CAD build for the part. Positions are in the model's coordinates, mm. Round coordinates to 2 decimals unless told otherwise and drop trailing zeros. Write each loop counter-clockwise with the first axis right and the second up, starting at its lowest first coordinate (ties: lowest second). Pieces come first, ordered by that corner, then holes. Notation, with made-up numbers: (18.25, 59) - (54.25, 59) arc R22 ccw to (54.25, 79) - close; hole circle Ø7 at (50.25, 9). An arc over 180 degrees is marked (long way). Answer in a Markdown table with one row per item.
```python
from build123d import *

# Parameters (mm, degrees)
SKETCH_3_R        = 1.65
EXTRUDE_242_DEPTH = 2
CHAMFER_C1_SIZE   = 1


with BuildPart() as part:
    # 草图3 → Extrude 242 (new body)
    with BuildSketch(Plane.XY):
        Polygon((-31, -60), (31, -60), (36, -50), (38, -45), (38, 50), (28, 66), (-28, 66), (-38, 50), (-38, -45), (-36, -50), align=None)
        with Locations((-22, -56)):
            Circle(SKETCH_3_R, mode=Mode.SUBTRACT)
        with Locations((-25, 53)):
            Circle(SKETCH_3_R, mode=Mode.SUBTRACT)
        with Locations((-34, -43)):
            Circle(SKETCH_3_R, mode=Mode.SUBTRACT)
        with Locations((-34, 43)):
            Circle(SKETCH_3_R, mode=Mode.SUBTRACT)
        with Locations((22, -56)):
            Circle(SKETCH_3_R, mode=Mode.SUBTRACT)
        with Locations((25, 53)):
            Circle(SKETCH_3_R, mode=Mode.SUBTRACT)
        with Locations((34, -43)):
            Circle(SKETCH_3_R, mode=Mode.SUBTRACT)
        with Locations((34, 43)):
            Circle(SKETCH_3_R, mode=Mode.SUBTRACT)
    extrude(amount=EXTRUDE_242_DEPTH)

    # 底盖全周向心倒角_C1
    # the kernel refuses this chamfer: 1 mm, written as the material it takes off along each edge
    with BuildSketch(Plane(origin=(-38.955099084, -42.612252289, 0), x_dir=(-0.02552928052838921, -0.010211712211355682, 0.9996219169112968), z_dir=(0.3713906763541037, -0.9284766908852594, 0)), Plane(origin=(35.044900916, -52.387747711, 0), x_dir=(0.025529280528384445, -0.010211712211353776, 0.9996219169112968), z_dir=(0.3713906763541037, 0.9284766908852594, 0))) as chamfer_c1_piece_1:
        Polygon((CHAMFER_C1_SIZE * 0.999621916911, -CHAMFER_C1_SIZE * 0.0274958766106), (-CHAMFER_C1_SIZE * 0.0274958766106, -CHAMFER_C1_SIZE * 0.999621916911), (0, 0), align=None)
    extrude(amount=10.528530783, mode=Mode.SUBTRACT)
    with BuildSketch(Plane(origin=(-38, 52.571682988, 0), x_dir=(-0.02749587661058908, 0, 0.9996219169112968), z_dir=(0, -1, 0)), Plane(origin=(38, -47.571682988, 0), x_dir=(0.02749587661058908, 0, 0.9996219169112968), z_dir=(0, 1, 0))) as chamfer_c1_piece_2:
        Polygon((CHAMFER_C1_SIZE * 0.999621916911, -CHAMFER_C1_SIZE * 0.0274958766106), (-CHAMFER_C1_SIZE * 0.0274958766106, -CHAMFER_C1_SIZE * 0.999621916911), (0, 0), align=None)
    extrude(amount=100.143365976, mode=Mode.SUBTRACT)
    with BuildSketch(Plane(origin=(-26.637010742, 68.180782812, 0), x_dir=(-0.023316456732911925, 0.014572785458069957, 0.9996219169112968), z_dir=(-0.52999894000318, -0.847998304005088, 0)), Plane(origin=(39.362989258, 47.819217188, 0), x_dir=(0.023316456732909444, 0.014572785458068402, 0.9996219169112968), z_dir=(-0.52999894000318, 0.847998304005088, 0))) as chamfer_c1_piece_3:
        Polygon((CHAMFER_C1_SIZE * 0.999621916911, -CHAMFER_C1_SIZE * 0.0274958766106), (-CHAMFER_C1_SIZE * 0.0274958766106, -CHAMFER_C1_SIZE * 0.999621916911), (0, 0), align=None)
    extrude(amount=24.01132824, mode=Mode.SUBTRACT)
    with BuildSketch(Plane(origin=(30.571682988, 66, 0), x_dir=(0, 0.027495876610582174, 0.9996219169112968), z_dir=(-1, 0, 0))) as chamfer_c1_piece_4:
        Polygon((CHAMFER_C1_SIZE * 0.999621916911, -CHAMFER_C1_SIZE * 0.0274958766106), (-CHAMFER_C1_SIZE * 0.0274958766106, -CHAMFER_C1_SIZE * 0.999621916911), (0, 0), align=None)
    extrude(amount=61.143365976, mode=Mode.SUBTRACT)
    with BuildSketch(Plane(origin=(29.849908404, -62.300183191, 0), x_dir=(0.02459305968088644, -0.01229652984044322, 0.9996219169112968), z_dir=(0.447213595499958, 0.894427190999916, 0)), Plane(origin=(-37.150091596, -47.699816809, 0), x_dir=(-0.024593059680886434, -0.012296529840443217, 0.9996219169112968), z_dir=(0.447213595499958, -0.894427190999916, 0))) as chamfer_c1_piece_5:
        Polygon((CHAMFER_C1_SIZE * 0.999621916911, -CHAMFER_C1_SIZE * 0.0274958766106), (-CHAMFER_C1_SIZE * 0.0274958766106, -CHAMFER_C1_SIZE * 0.999621916911), (0, 0), align=None)
    extrude(amount=16.323705863, mode=Mode.SUBTRACT)
    with BuildSketch(Plane(origin=(-33.571682988, -60, 0), x_dir=(0, -0.02749587661058908, 0.9996219169112968), z_dir=(1, 0, 0))) as chamfer_c1_piece_6:
        Polygon((CHAMFER_C1_SIZE * 0.999621916911, -CHAMFER_C1_SIZE * 0.0274958766106), (-CHAMFER_C1_SIZE * 0.0274958766106, -CHAMFER_C1_SIZE * 0.999621916911), (0, 0), align=None)
    extrude(amount=67.143365976, mode=Mode.SUBTRACT)


solid = part.part
```
Q1. Saw through at A-A on x = -22. List the corners of the cut face in (y, z).
Computed:
| item | result |
|---|---|
| outline | (-60, 1) - (-59, 0) - (-57.65, 0) - (-57.65, 2) - (-60, 2) - close; (-54.35, 0) - (65, 0) - (66, 1) - (66, 2) - (-54.35, 2) - close |
Q2. Flat gauge pin, fed straight in: pin 1 (2 mm diameter, centred on x = -22, y = -56, fed in from -Z). Where does the tip first touch, or does it go through?
Computed:
| item | result |
|---|---|
| pin 1 | passes through |
Q3. Drill centre lines: line 1 (Y direction, x = 23.5, z = 0.25); line 2 (Y direction, x = -25, z = 1); line 3 (Y direction, x = -24, z = 0.8). Where is each one in solid material? Low to high.
Computed:
| item | result |
|---|---|
| line 1 | y = -59.25 to -56.69, -55.31 to 52.31, 53.69 to 65.25 |
| line 2 | y = -60 to 51.35, 54.65 to 66 |
| line 3 | y = -59.8 to 51.69, 54.31 to 65.8 |
Q4. Saw through at B-B on y = 43. List the corners of the cut face in (x, z).
Computed:
| item | result |
|---|---|
| outline | (-38, 1) - (-37, 0) - (-35.65, 0) - (-35.65, 2) - (-38, 2) - close; (-32.35, 0) - (32.35, 0) - (32.35, 2) - (-32.35, 2) - close; (35.65, 0) - (37, 0) - (38, 1) - (38, 2) - (35.65, 2) - close |
Q5. Saw through at D-D on y = -56. List the corners of the cut face in (x, z).
Computed:
| item | result |
|---|---|
| outline | (-33, 1) - (-31.88, 0) - (-23.65, 0) - (-23.65, 2) - (-33, 2) - close; (-20.35, 0) - (20.35, 0) - (20.35, 2) - (-20.35, 2) - close; (23.65, 0) - (31.88, 0) - (33, 1) - (33, 2) - (23.65, 2) - close |
Q6. Pull direction X, two halves, no side cores. Call faces 1 (the cylindrical face through (-26.65, 53.07, 0.99)), 2 (the flat face through (33.465, -55.07, 1.493)), 3 (the flat face through (-32.93, 58.11, 1.49)): released by +X, released by -X, zero draft, split by the parting line, or undercut.
Computed:
| item | result |
|---|---|
| face 1 | undercut |
| face 2 | released by +X |
| face 3 | released by -X |
Q7. Saw through at C-C on z = 1.3. Count the separate pieces of the cut face and the enclosed holes in it, then the cut area to 3 significant figures.
Computed:
| item | result |
|---|---|
| separate pieces | 1 |
| enclosed holes | 8 |
| area | 9,250 mm2 |
